Solid Edge part; units mm, degrees
sketch "Sketch1" plane through (0, 0, 0) normal (0, -1, 0) x (1, 0, 0)
  line L0 (-45, -40) -> (45, -40)
  line L1 (45, -40) -> (45, 40)
  line L2 (45, 40) -> (-45, 40)
  line L3 (-45, 40) -> (-45, -40)
  dimension "D1" = 45
  dimension "D2" = 45
extrude "Protrusion1" add sketch "Sketch1" against normal blind 10
sketch "Sketch2" plane through (0, 0, 0) normal (0, -1, 0) x (1, 0, 0)
  circle A0 centre (-40, 30) radius 1.4
  circle A1 centre (-40, -30) radius 1.4
  circle A2 centre (40, -30) radius 1.4
  circle A3 centre (40, 30) radius 1.4
  dimension "D1" = 40
  dimension "D2" = 40
extrude "Cutout1" cut sketch "Sketch2" against normal through all
sketch "Sketch3" plane through (0, 0, 0) normal (0, -1, 0) x (1, 0, 0)
  circle A0 centre (-21, 16) radius 4
  circle A1 centre (-21, -16) radius 4
  circle A2 centre (21, -16) radius 4
  circle A3 centre (21, 16) radius 4
extrude "Extrusionsausschnitt_2" cut sketch "Sketch3" against normal blind 5
sketch "Sketch4" plane through (0, 0, 0) normal (0, -1, 0) x (1, 0, 0)
  circle A0 centre (-21, 16) radius 1.75
  circle A1 centre (-21, -16) radius 1.75
  circle A2 centre (21, -16) radius 1.75
  circle A3 centre (21, 16) radius 1.75
extrude "Cutout2" cut sketch "Sketch4" against normal through all
fillet "Verrundung_1" radius 4 4 edges at (-45, 5, 40) (45, 5, 40) (45, 5, -40) (-45, 5, -40)
chamfer "Fase_1" distance 0.5 angle 60 4 edges at (38.6, 0, 30) (-41.4, 0, 30) (-41.4, 0, -30) (38.6, 0, -30) measured on face at (-29.1, 0, 27.4667)
chamfer "Fase_2" distance 0.5 angle 60 4 edges at (-40, 10, 31.4) (40, 10, 31.4) (40, 10, -28.6) (-40, 10, -28.6) measured on face at (-29.1, 10, 27.4667)
chamfer "Fase_3" distance 0.5 angle 60 4 edges at (-21, 10, 17.75) (21, 10, 17.75) (-21, 10, -14.25) (21, 10, -14.25) measured on face at (-29.1, 10, 27.4667)
chamfer "Fase_4" distance 0.5 angle 60 4 edges at (-21, 5, 14.25) (-21, 5, -17.75) (21, 5, 14.25) (21, 5, -17.75) measured on face at (-23.5867, 5, 18.7467) measured on face at (18.4133, 5, 18.7467) measured on face at (-23.5867, 5, -13.2533) measured on face at (18.4133, 5, -13.2533)
properties material "Nylon, allgemein"
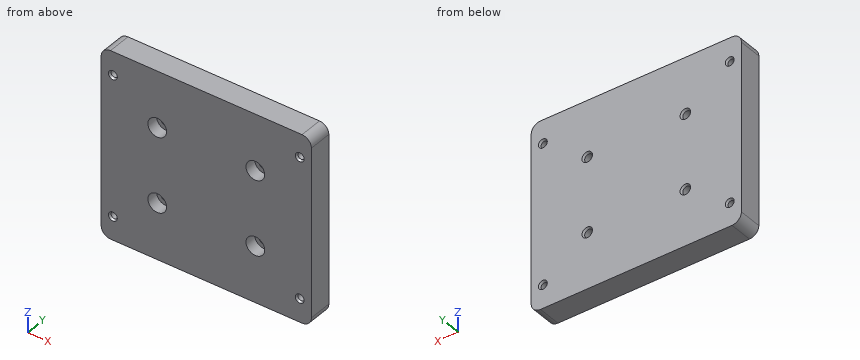
Work out the finished part from the listing and answer in its coordinate system (mm). Round coordinates to 2 decimals unless told otherwise and drop trailing zeros. Loops run counter-clockwise (first coordinate to the right, second up) from the corner with the lowest first, then second, coordinate; pieces in that order, holes last.
(1) Find the intervals of material crossed by L1, parallel to Z at x = -40, y = 4.25; L2, parallel to Z at x = -40.5, y = 3.75, in increasing order.
Computed values:
L1: z = -40 to -31.4, -28.6 to 28.6, 31.4 to 40
L2: z = -40 to -31.31, -28.69 to 28.69, 31.31 to 40
(2) The part is cut by section B-B, the plane x = 40. Give the vertices of the cut face in (y, z).
Computed values:
outline: (0, -40) - (10, -40) - (10, -31.9) - (9.13, -31.4) - (0.87, -31.4) - (0, -31.9) - close; (0, -28.1) - (0.87, -28.6) - (9.13, -28.6) - (10, -28.1) - (10, 28.1) - (9.13, 28.6) - (0.87, 28.6) - (0, 28.1) - close; (0, 31.9) - (0.87, 31.4) - (9.13, 31.4) - (10, 31.9) - (10, 40) - (0, 40) - close
(3) The part is cut by section A-A, the plane z = -30. Give the vertices of the cut face in (x, y), and give its area (3 significant figures).
Computed values:
outline: (-45, 0) - (-41.9, 0) - (-41.4, 0.87) - (-41.4, 9.13) - (-41.9, 10) - (-45, 10) - close; (-38.6, 0.87) - (-38.1, 0) - (38.1, 0) - (38.6, 0.87) - (38.6, 9.13) - (38.1, 10) - (-38.1, 10) - (-38.6, 9.13) - close; (41.4, 0.87) - (41.9, 0) - (45, 0) - (45, 10) - (41.9, 10) - (41.4, 9.13) - close
area: 842 mm2
(4) The part is cut by section C-C, the plane z = -16. Give the vertices of the cut face in (x, y), and give its area (3 significant figures).
Computed values:
outline: (-45, 0) - (-25, 0) - (-25, 5) - (-23.25, 5) - (-22.75, 5.87) - (-22.75, 9.13) - (-23.25, 10) - (-45, 10) - close; (-19.25, 5.87) - (-18.75, 5) - (-17, 5) - (-17, 0) - (17, 0) - (17, 5) - (18.75, 5) - (19.25, 5.87) - (19.25, 9.13) - (18.75, 10) - (-18.75, 10) - (-19.25, 9.13) - close; (22.75, 5.87) - (23.25, 5) - (25, 5) - (25, 0) - (45, 0) - (45, 10) - (23.25, 10) - (22.75, 9.13) - close
area: 783 mm2
(5) The part is cut by section D-D, the plane x = -21. Give the vertices of the cut face in (y, z), and give its area (3 significant figures).
Computed values:
outline: (0, -40) - (10, -40) - (10, -18.25) - (9.13, -17.75) - (5.87, -17.75) - (5, -18.25) - (5, -20) - (0, -20) - close; (0, -12) - (5, -12) - (5, -13.75) - (5.87, -14.25) - (9.13, -14.25) - (10, -13.75) - (10, 13.75) - (9.13, 14.25) - (5.87, 14.25) - (5, 13.75) - (5, 12) - (0, 12) - close; (0, 20) - (5, 20) - (5, 18.25) - (5.87, 17.75) - (9.13, 17.75) - (10, 18.25) - (10, 40) - (0, 40) - close
area: 683 mm2
(6) Each of these flat-tipped pins is pushed along its axis until it touches: P1, Ø10.5, axis at x = 21, z = 16, coming from the +Y side; P2, Ø5.5, axis at x = -21, z = -16, coming from the -Y side; P3, Ø4, axis at x = -21, z = 16, coming from the -Y side; P4, Ø2, axis at x = -40, z = -30, coming from the -Y side. Where does it stop, or does it pass through?
Computed values:
P1: stops at y = 10
P2: stops at y = 5
P3: stops at y = 5.43
P4: passes through
